Design review of the part built by this model. Coordinates are the model's own, in mm. A direction names the side the tool comes from. Give positions to 0.01 mm unless a question says otherwise; leave off trailing zeros. Write each loop counter-clockwise with the first axis right and the second up, starting at its lowest first coordinate (ties: lowest second). Pieces come first, ordered by that corner, then holes.
Autodesk Inventor part; units mm, degrees
ref_plane "YZ Plane" through (0, 0, 0) normal (1, 0, 0) x (0, 1, 0)
ref_plane "XZ Plane" through (0, 0, 0) normal (0, 1, 0) x (-1, 0, 0)
ref_plane "XY Plane" through (0, 0, 0) normal (0, 0, 1) x (1, 0, 0)
sketch "Sketch1" plane through (0, 0, 0) normal (0, 1, 0) x (-1, 0, 0)
  line L0 (0, 0) -> (-82.55, 0)
  line L1 (-82.55, 0) -> (-82.55, 38.1)
  line L2 (-82.55, 38.1) -> (0, 38.1)
  line L3 (0, 38.1) -> (0, 0)
  dimension "d0" = 82.55
  dimension "d1" = 38.1
extrude "Extrusion1" add sketch "Sketch1" along normal blind 3.175
sketch "Sketch2" plane through (0, 3.175, 0) normal (0, 1, 0) x (1, 0, 0)
  line L0 (82.55, 0) -> (0, 0)
  line L1 (0, 0) -> (0, -38.1)
  line L2 (0, -38.1) -> (82.55, -38.1)
  line L3 (82.55, -38.1) -> (82.55, 0)
  line L4 (0, -36.5125) -> (82.55, -36.5125)
  line L5 (82.55, -36.5125) -> (82.55, -33.3121)
  line L6 (82.55, -33.3121) -> (0, -33.3121)
  line L7 (0, -33.3121) -> (0, -36.5125)
  line L8 (1.5875, -3.175) -> (80.9625, -3.175)
  line L9 (80.9625, -3.175) -> (80.9625, -6.604)
  line L10 (80.9625, -6.604) -> (1.5875, -6.604)
  line L11 (1.5875, -6.604) -> (1.5875, -3.175)
  dimension "d6" = 3.2004
  dimension "d7" = 1.5875
  dimension "d10" = 3.175
  dimension "d11" = 3.429
  dimension "d12" = 1.5875
  dimension "d13" = 1.5875
extrude "Extrusion2" cut sketch "Sketch2" against normal blind 1.5875 contours L3 L4 L1 L6
sketch "Sketch3" plane through (0, 3.175, 0) normal (0, 1, 0) x (1, 0, 0)
  line L0 (82.55, -33.3121) -> (82.55, 0)
  line L1 (82.55, 0) -> (0, 0)
  line L2 (0, 0) -> (0, -33.3121)
  line L3 (1.5875, -3.175) -> (80.9625, -3.175)
  line L4 (80.9625, -3.175) -> (80.9625, -6.604)
  line L5 (80.9625, -6.604) -> (1.5875, -6.604)
  line L6 (1.5875, -6.604) -> (1.5875, -3.175)
  dimension "d14" = 1.5875
  dimension "d15" = 1.5875
  dimension "d16" = 3.175
  dimension "d17" = 3.429
extrude "Extrusion3" cut sketch "Sketch3" against normal blind 1.5875
sketch "Sketch4" plane through (0, 3.175, 0) normal (0, 1, 0) x (1, 0, 0)
  line L0 (0, -38.1) -> (1.5875, -38.1)
  line L1 (1.5875, -38.1) -> (1.5875, -31.75)
  line L2 (1.5875, -31.75) -> (0, -31.75)
  line L3 (0, -31.75) -> (0, -38.1)
  line L4 (82.55, -38.1) -> (80.9625, -38.1)
  line L5 (80.9625, -38.1) -> (80.9625, -31.75)
  line L6 (80.9625, -31.75) -> (82.55, -31.75)
  line L7 (82.55, -31.75) -> (82.55, -38.1)
  point P0 (0, 0)
  dimension "d20" = 1.5875
  dimension "d21" = 6.35
  dimension "d22" = 6.35
  dimension "d23" = 1.5875
extrude "Extrusion4" cut sketch "Sketch4" against normal blind 25.4
fillet "Fillet1" radius 1.5875 1 edges at (80.9625, 1.5875, 31.75)
fillet "Fillet2" radius 1.5875 1 edges at (1.5875, 1.5875, 31.75)
properties part number "Electronics Container Part 4"
(1) Consider section A-A, the plane y = 2.35. Give the number of separate pieces and of enclosed holes in the cut face, then the cut area to 3 significant figures.
Resolved:
separate pieces: 2
enclosed holes: 1
area: 2,600 mm2
(2) Clearance check with flat-ended pins moving along their axes: P1, Ø1.7, axis at x = 32, z = 5.5, coming from the +Y side; P2, Ø1.6, axis at y = 2, z = 35.5, coming from the -X side. State where each tip first meets the part, or that it passes through.
Resolved:
P1: stops at y = 1.59
P2: stops at x = 1.59
(3) Consider section B-B, the plane x = 15. Give the boundary of the cut face in (y, z) (1 decimal), then the cut area to 3 significant figures.
Resolved:
outline: (0, 0) - (3.2, 0) - (3.2, 3.2) - (1.6, 3.2) - (1.6, 6.6) - (3.2, 6.6) - (3.2, 33.3) - (1.6, 33.3) - (1.6, 36.5) - (3.2, 36.5) - (3.2, 38.1) - (0, 38.1) - close
area: 110 mm2
(4) To check wall thickness, follow L1, parallel to Z at x = 37.5, y = 2.55 (1 decimal); L2, parallel to X at y = 1.8, z = 6; L3, parallel to X at y = 0.25, z = 34. State the ranges of each line that lie inside material, in increasing order.
Resolved:
L1: z = 0 to 3.2, 6.6 to 33.3, 36.5 to 38.1
L2: x = 0 to 1.59, 80.96 to 82.55
L3: x = 1.59 to 80.96
(5) Tool access review of faces 5 (the face through (82.55, 2, 16)), 6 (the face through (41, 1.588, 5)), 7 (the face through (1.588, 1, 36)), 8 (the face through (42, 2, 33.312)): name each direction out of +Z, -Z, +X, -X, +Y, -Y from which nothing blocks a thin tool from reaching the whole face with its end or side.
Resolved:
face 5: +Z, -Z, +X, +Y, -Y
face 6: +Y
face 7: +Z, -X, +Y, -Y
face 8: +X, -X, +Y
(6) Consider section C-C, the plane z = 34.5. Give the boundary of the cut face in (x, y).
Resolved:
outline: (1.59, 0) - (80.96, 0) - (80.96, 1.59) - (1.59, 1.59) - close
(7) Mouldability with a two-part tool opening along X and no side actions: class faces 1 (the face through (1.588, 2, 5)), 2 (the face through (42, 3.175, 17)), 3 (the face through (80.962, 1, 36)), 4 (the face through (1.11, 1.57, 32.2)) as pulls with the +X half, pulls with the -X half, needs draft (parallel to the pull), parting line crosses it, or undercut.
Resolved:
face 1: undercut
face 2: needs draft
face 3: pulls with the +X half
face 4: pulls with the -X half
